Read the model definition and answer for the solid it produces. Units are mm, in the model's axes. A direction names the side the tool comes from. Coordinates: 2 decimals unless noted, no trailing zeros. Loops run counter-clockwise (first coordinate to the right, second up) from the corner with the lowest first, then second, coordinate; pieces in that order, holes last.
from build123d import *

# Parameters (mm, degrees)
SKETCH1_R      = 27
RING_DEPTH     = 20
SKETCH2_W      = 58
SKETCH2_H      = 4
FLATS_DEPTH    = 14
SKETCH3_R      = 22.5
BORE_DEPTH     = 20
SKETCH4_R      = 24.5
BORE_LOW_DEPTH = 10
TEETH_DEPTH    = 10


with BuildPart() as part:
    # Sketch1 → Ring (new body)
    with BuildSketch(Plane.XY):
        Circle(SKETCH1_R)
    extrude(amount=RING_DEPTH)

    # Sketch2 → Flats (cut)
    with BuildSketch(Plane.XY.offset(6)):
        with Locations((0, 27)):
            Rectangle(SKETCH2_W, SKETCH2_H)
        with Locations((0, -27)):
            Rectangle(SKETCH2_W, SKETCH2_H)
    extrude(amount=FLATS_DEPTH, mode=Mode.SUBTRACT)

    # Sketch3 → Bore (cut)
    with BuildSketch(Plane.XY):
        Circle(SKETCH3_R)
    extrude(amount=BORE_DEPTH, mode=Mode.SUBTRACT)

    # Sketch4 → Bore_low (cut)
    with BuildSketch(Plane.XY):
        Circle(SKETCH4_R)
    extrude(amount=BORE_LOW_DEPTH, mode=Mode.SUBTRACT)

    # Sketch5 → Teeth (cut)
    with BuildSketch(Plane.XY.offset(10)):
        Polygon((24.5, 0), (21.5, 3), (21.5, -3), align=None)
        Polygon((23.300884649, 7.570916362), (19.520664117, 9.497034928), (21.374766083, 3.79069583), align=None)
        Polygon((19.820916362, 14.400738681), (15.630509622, 15.064433907), (19.157221136, 10.210331941), align=None)
        Polygon((14.400738681, 19.820916362), (10.210331941, 19.157221136), (15.064433907, 15.630509622), align=None)
        Polygon((7.570916362, 23.300884649), (3.79069583, 21.374766083), (9.497034928, 19.520664117), align=None)
        Polygon((0, 24.5), (-3, 21.5), (3, 21.5), align=None)
        Polygon((-7.570916362, 23.300884649), (-9.497034928, 19.520664117), (-3.79069583, 21.374766083), align=None)
        Polygon((-14.400738681, 19.820916362), (-15.064433907, 15.630509622), (-10.210331941, 19.157221136), align=None)
        Polygon((-19.820916362, 14.400738681), (-19.157221136, 10.210331941), (-15.630509622, 15.064433907), align=None)
        Polygon((-23.300884649, 7.570916362), (-21.374766083, 3.79069583), (-19.520664117, 9.497034928), align=None)
        Polygon((-24.5, 0), (-21.5, -3), (-21.5, 3), align=None)
        Polygon((-23.300884649, -7.570916362), (-19.520664117, -9.497034928), (-21.374766083, -3.79069583), align=None)
        Polygon((-19.820916362, -14.400738681), (-15.630509622, -15.064433907), (-19.157221136, -10.210331941), align=None)
        Polygon((-14.400738681, -19.820916362), (-10.210331941, -19.157221136), (-15.064433907, -15.630509622), align=None)
        Polygon((-7.570916362, -23.300884649), (-3.79069583, -21.374766083), (-9.497034928, -19.520664117), align=None)
        Polygon((0, -24.5), (3, -21.5), (-3, -21.5), align=None)
        Polygon((7.570916362, -23.300884649), (9.497034928, -19.520664117), (3.79069583, -21.374766083), align=None)
        Polygon((14.400738681, -19.820916362), (15.064433907, -15.630509622), (10.210331941, -19.157221136), align=None)
        Polygon((19.820916362, -14.400738681), (19.157221136, -10.210331941), (15.630509622, -15.064433907), align=None)
        Polygon((23.300884649, -7.570916362), (21.374766083, -3.79069583), (19.520664117, -9.497034928), align=None)
    extrude(amount=TEETH_DEPTH, mode=Mode.SUBTRACT)


solid = part.part
Item 1: A cutting plane is placed at D-D on x = -4. Determine the outline of the cut face in (y, z).
Numbers:
outline: (-26.7, 0) - (-24.17, 0) - (-24.17, 10) - (-22.14, 10) - (-22.14, 20) - (-25, 20) - (-25, 6) - (-26.7, 6) - close; (22.14, 10) - (24.17, 10) - (24.17, 0) - (26.7, 0) - (26.7, 6) - (25, 6) - (25, 20) - (22.14, 20) - close
Item 2: A cutting plane is placed at C-C on z = 7.25. Determine the outline of the cut face in (x, y), then the cut area to 3 significant figures.
Numbers:
outline: (-10.2, -25) - (10.2, -25) arc R27 ccw to (10.2, 25) - (-10.2, 25) arc R27 ccw to start; hole circle Ø49 at (0, 0)
area: 350 mm2
Item 3: A cutting plane is placed at A-A on y = -16. Determine the outline of the cut face in (x, z).
Numbers:
outline: (-21.75, 0) - (-18.55, 0) - (-18.55, 10) - (-15.82, 10) - (-15.82, 20) - (-21.75, 20) - close; (15.82, 10) - (18.55, 10) - (18.55, 0) - (21.75, 0) - (21.75, 20) - (15.82, 20) - close
Item 4: Determine the mould class of faces 1 (the face through (0, -25, 13)), 2 (the face through (-17, 17, 10)) for opening direction X: released by +X, released by -X, zero draft, split by the parting line, or undercut.
Numbers:
face 1: zero draft
face 2: undercut
Item 5: Given pin 1 (1.6 mm diameter, centred on x = 1, y = -26, fed in from +Z); pin 2 (1.5 mm diameter, centred on y = -7, z = 4, fed in from -X); pin 3 (1.2 mm diameter, centred on x = 10.5, y = 21, fed in from -Z), each flat-ended and moving along its own axis, determine where each tip first touches the part or whether it passes through.
Numbers:
pin 1: stops at z = 6
pin 2: stops at x = -26.27
pin 3: stops at z = 10
Item 6: A cutting plane is placed at B-B on x = 13.5. Determine the outline of the cut face in (y, z).
Numbers:
outline: (-23.38, 0) - (-20.45, 0) - (-20.45, 10) - (-19.68, 10) - (-19.68, 20) - (-23.38, 20) - close; (19.68, 10) - (20.45, 10) - (20.45, 0) - (23.38, 0) - (23.38, 20) - (19.68, 20) - close
Item 7: Which of the six approach directions +Z, -Z, +X, -X, +Y, -Y give full straight-line access (tool end or side, diameter ignored) to faces 3 (the face through (22.618, 6.231, 14.93)), 4 (the face through (23, -4, 10))?
Numbers:
face 3: +Z, -Z
face 4: -Z
Item 8: Find the intervals of material crossed by line 1 along Y through (x, z) = (0, 3); line 2 along Y through (x, z) = (0, 6.25), in increasing order.
Numbers:
line 1: y = -27 to -24.5, 24.5 to 27
line 2: y = -25 to -24.5, 24.5 to 25
